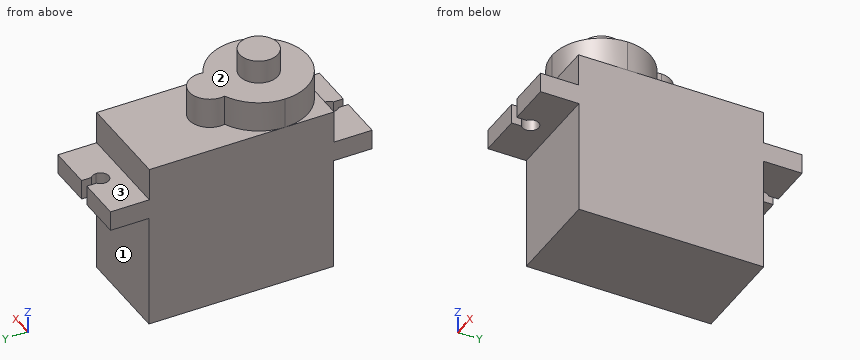
from build123d import *

# Parameters (mm, degrees)
F0_W     = 12
F0_H     = 22.6
F1_DEPTH = 14
F2_W     = 12
F2_H     = 22.6
F3_DEPTH = 2.45
F4_W     = 12
F4_H     = 22.6
F5_DEPTH = 4
F7_DEPTH = 3.74
F8_R     = 2.335
F9_DEPTH = 2.9


# Not quite as in the source:
# - a feature names something its author has since deleted; it is built from what else it names


with BuildPart() as f1:
    # F0 (on Top) → F1 (new body)
    with BuildSketch(Plane.XY):
        with Locations((13.4373875856, -22.2866622627)):
            Rectangle(F0_W, F0_H)
    extrude(amount=F1_DEPTH)

    # F2 (on face) → F3 (join)
    with BuildSketch(Plane.XY.offset(14)):
        with BuildLine():
            Line((7.4373875856, -10.9866622627), (19.4373875856, -10.9866622627))
            Line((19.4373875856, -10.9866622627), (19.4373875856, -6.2866622627))
            Line((19.4373875856, -6.2866622627), (14.0248552029, -6.2866622627))
            Line((14.0248552029, -6.2866622627), (14.0248552029, -7.4774145882))
            ThreePointArc((14.0248552029, -7.4774145882), (14.3283049828, -7.8324968838), (14.4373875856, -8.2866622627))
            ThreePointArc((14.4373875856, -8.2866622627), (12.9832222068, -9.1775796599), (12.8499199684, -7.4774145882))
            Line((12.8499199684, -7.4774145882), (12.8499199684, -6.2866622627))
            Line((12.8499199684, -6.2866622627), (7.4373875856, -6.2866622627))
            Line((7.4373875856, -6.2866622627), (7.4373875856, -10.9866622627))
        make_face()
        with BuildLine():
            Line((19.4373875856, -38.2866622627), (19.4373875856, -33.5866622627))
            Line((19.4373875856, -33.5866622627), (7.4373875856, -33.5866622627))
            Line((7.4373875856, -33.5866622627), (7.4373875856, -38.2866622627))
            Line((7.4373875856, -38.2866622627), (12.8499199684, -38.2866622627))
            Line((12.8499199684, -38.2866622627), (12.8499199684, -37.0959099372))
            ThreePointArc((12.8499199684, -37.0959099372), (12.9832222068, -35.3957448655), (14.4373875856, -36.2866622627))
            ThreePointArc((14.4373875856, -36.2866622627), (14.3283049828, -36.7408276416), (14.0248552029, -37.0959099372))
            Line((14.0248552029, -37.0959099372), (14.0248552029, -38.2866622627))
            Line((14.0248552029, -38.2866622627), (19.4373875856, -38.2866622627))
        make_face()
        with Locations((13.4373875856, -22.2866622627)):
            Rectangle(F2_W, F2_H)
    extrude(amount=F3_DEPTH)

    # F4 (on face) → F5 (join)
    with BuildSketch(Plane.XY.offset(16.45)):
        with Locations((13.4373875856, -22.3371585727)):
            Rectangle(F4_W, F4_H)
    extrude(amount=F5_DEPTH)

    # F6 (on face) → F7 (join)
    with BuildSketch(Plane.XY.offset(20.45)):
        with BuildLine():
            ThreePointArc((13.4373875856, -33.6371585727), (17.6800282728, -31.8797992598), (19.4373875856, -27.6371585727))
            ThreePointArc((19.4373875856, -27.6371585727), (18.4708192303, -24.371493881), (15.8825322928, -22.157991906))
            ThreePointArc((15.8825322928, -22.157991906), (13.4373875856, -24.1371585727), (10.9922428785, -22.157991906))
            ThreePointArc((10.9922428785, -22.157991906), (8.403955941, -24.371493881), (7.4373875856, -27.6371585727))
            ThreePointArc((7.4373875856, -27.6371585727), (9.1947468985, -31.8797992598), (13.4373875856, -33.6371585727))
        make_face()
        with BuildLine():
            ThreePointArc((10.9922428785, -22.157991906), (13.4373875856, -24.1371585727), (15.8825322928, -22.157991906))
            ThreePointArc((15.8825322928, -22.157991906), (13.4373875856, -21.6371585727), (10.9922428785, -22.157991906))
        make_face()
        with BuildLine():
            ThreePointArc((10.9922428785, -22.157991906), (13.4373875856, -21.6371585727), (15.8825322928, -22.157991906))
            ThreePointArc((15.8825322928, -22.157991906), (15.9236359409, -21.8990156254), (15.9373875856, -21.6371585727))
            ThreePointArc((15.9373875856, -21.6371585727), (13.1755305329, -19.1509102174), (10.9922428785, -22.157991906))
        make_face()
    extrude(amount=F7_DEPTH)

    # F8 (on face) → F9 (join)
    with BuildSketch(Plane.XY.offset(24.19)):
        with Locations((13.4373875856, -27.6371585727)):
            Circle(F8_R)
    extrude(amount=F9_DEPTH)


solid = f1.part
Part model, mm, in its own coordinate system. Face numbers are marked on the shaded views. A direction names the side the tool comes from. Give positions to 0.01 mm unless a question says otherwise; leave off trailing zeros. Loops run counter-clockwise (first coordinate to the right, second up) from the corner with the lowest first, then second, coordinate; pieces in that order, holes last. Notation, with made-up numbers: M -4,58 L 54,58 A31 cw 54,91 Z; hole C 89,-19 d4. An arc over 180 degrees is marked long. Put each result on its own line as item: value. Start each with the question number.
1) Saw through at D-D (y = -33). List the corners of the cut face in (x, z), then the cut area to 3 significant figures.
2) Probe probe 1 along Z at (x, y) = (16.25, -25.5); probe 2 along Z at (x, y) = (14.25, -18); probe 3 along Y at (x, z) = (15, 20). List the from-to ranges inside material, lowest first.
3) 3-axis set-ups, long thin cutter, end or side, ignore diameter. For the marked faces 1, 2 and 3: which of +Z, -Z, +X, -X, +Y, -Y reach the whole face in a straight line?
4) Saw through at C-C (x = 15). List the corners of the cut face in (y, z), then the cut area to 3 significant figures.
5) Saw through at B-B (z = 21.25). List the corners of the cut face in (x, y).
6) Flat gauge pins, fed straight in: pin 1 (1 mm diameter, centred on x = 13.5, z = 10, fed in from -Y); pin 2 (1.4 mm diameter, centred on x = 12.5, y = -10, fed in from -Z); pin 3 (6 mm diameter, centred on x = 10.5, y = -28, fed in from +Z); pin 4 (3 mm diameter, centred on x = 16.5, y = -30, fed in from +Z). Where does each tip first touch, or does it go through?
Numbers:
1. outline: M 7.44,0 L 19.44,0 L 19.44,20.45 L 16.13,20.45 L 16.13,24.19 L 10.75,24.19 L 10.75,20.45 L 7.44,20.45 Z
1. area: 266 mm^2
2. probe 1: 0 to 24.19
2. probe 2: 0 to 20.45
2. probe 3: -33.64 to -11.04
3. face 1: -Z, +X, -X, +Y
3. face 2: +Z
3. face 3: +Z, +X, -X, +Y
4. outline: M -38.29,14 L -33.59,14 L -33.59,0 L -10.99,0 L -10.99,14 L -6.29,14 L -6.29,16.45 L -11.04,16.45 L -11.04,20.45 L -19.69,20.45 L -19.69,24.19 L -25.9,24.19 L -25.9,27.09 L -29.37,27.09 L -29.37,24.19 L -33.43,24.19 L -33.43,20.45 L -33.64,20.45 L -33.64,16.45 L -38.29,16.45 Z
4. area: 547 mm^2
5. outline: M 10.99,-22.16 A6 ccw long 15.88,-22.16 A2.5 ccw long Z
6. pin 1: y = -33.59
6. pin 2: z = 14
6. pin 3: z = 27.09
6. pin 4: z = 24.19
